Read the model definition and answer for the solid it produces. Units are mm, in the model's axes. Face numbers are marked on the shaded views. A direction names the side the tool comes from. Coordinates: 2 decimals unless noted, no trailing zeros. Write each loop counter-clockwise with the first axis right and the second up, starting at its lowest first coordinate (ties: lowest second). Pieces come first, ordered by that corner, then holes. Notation, with made-up numbers: (-14, 82) - (33, 82) arc R13 ccw to (33, 95) - close; hole circle Ø11 at (11, 88.25). An arc over 180 degrees is marked (long way). Use a Markdown table: item, result.
from build123d import *

# Parameters (mm, degrees)
SKETCH1_R           = 1.65
BOSS_EXTRUDE1_DEPTH = 2
BOSS_EXTRUDE2_DEPTH = 18
SKETCH3_W           = 13
SKETCH3_H           = 10
BOSS_EXTRUDE3_DEPTH = 10
SKETCH4_R           = 3.25
CUT_EXTRUDE1_DEPTH  = 10
CIRPATTERN1_COUNT   = 3


with BuildPart() as part:
    # Sketch1 → Boss-Extrude1 (new body)
    with BuildSketch(Plane(origin=(0, 0, 0), x_dir=(1, 0, 0), z_dir=(0, 1, 0))):
        with BuildLine():
            Line((14.5, 47.85133227), (48.690469351, -11.36829778))
            ThreePointArc((48.690469351, -11.36829778), (43.301270189, -25), (34.190469351, -36.48303449))
            Line((34.190469351, -36.48303449), (-34.190469351, -36.48303449))
            ThreePointArc((-34.190469351, -36.48303449), (-43.301270189, -25), (-48.690469351, -11.36829778))
            Line((-48.690469351, -11.36829778), (-14.5, 47.85133227))
            ThreePointArc((-14.5, 47.85133227), (0, 50), (14.5, 47.85133227))
        make_face()
        with Locations(Location((0, 45, 0), (0, 0, 270))):
            Circle(SKETCH1_R, mode=Mode.SUBTRACT)
        with Locations(Location((38.97114317, -22.5, 0), (0, 0, 270))):
            Circle(SKETCH1_R, mode=Mode.SUBTRACT)
        with Locations(Location((-38.97114317, -22.5, 0), (0, 0, 270))):
            Circle(SKETCH1_R, mode=Mode.SUBTRACT)
    extrude(amount=BOSS_EXTRUDE1_DEPTH)

    # Sketch2 → Boss-Extrude2 (add)
    with BuildSketch(Plane(origin=(0, 2, 0), x_dir=(1, 0, 0), z_dir=(0, 1, 0))):
        with BuildLine():
            Line((-14.5, 47.85133227), (-14.5, 8.371578903))
            Line((-14.5, 8.371578903), (-48.690469351, -11.36829778))
            ThreePointArc((-48.690469351, -11.36829778), (-48.443824061, -12.377233549), (-48.176274578, -13.380828366))
            Line((-48.176274578, -13.380828366), (-12.5, 7.216878365))
            Line((-12.5, 7.216878365), (-12.5, 48.412291828))
            ThreePointArc((-12.5, 48.412291828), (-13.502913349, 48.142199068), (-14.5, 47.85133227))
        make_face()
        with BuildLine():
            Line((14.5, 47.85133227), (14.5, 8.371578903))
            Line((14.5, 8.371578903), (48.690469351, -11.36829778))
            ThreePointArc((48.690469351, -11.36829778), (48.443824061, -12.377233549), (48.176274578, -13.380828366))
            Line((48.176274578, -13.380828366), (12.5, 7.216878365))
            Line((12.5, 7.216878365), (12.5, 48.412291828))
            ThreePointArc((12.5, 48.412291828), (13.502913349, 48.142199068), (14.5, 47.85133227))
        make_face()
        with BuildLine():
            Line((-34.190469351, -36.48303449), (0, -16.743157806))
            Line((0, -16.743157806), (34.190469351, -36.48303449))
            ThreePointArc((34.190469351, -36.48303449), (34.940910712, -35.764965519), (35.676274578, -35.031463461))
            Line((35.676274578, -35.031463461), (0, -14.43375673))
            Line((0, -14.43375673), (-35.676274578, -35.031463461))
            ThreePointArc((-35.676274578, -35.031463461), (-34.940910712, -35.764965519), (-34.190469351, -36.48303449))
        make_face()
    extrude(amount=BOSS_EXTRUDE2_DEPTH)

    # Sketch3 → Boss-Extrude3 (add)
    with BuildSketch(Plane(origin=(31.595234675, 0, -18.241517245), x_dir=(-0.5000000000000003, 0, -0.8660254037844386), z_dir=(0.8660254037844385, 0, -0.5000000000000002))):
        with Locations((0, 7)):
            Rectangle(SKETCH3_W, SKETCH3_H)
    boss_extrude3 = extrude(amount=-BOSS_EXTRUDE3_DEPTH)

    # Sketch4 → Cut-Extrude1 (cut)
    with BuildSketch(Plane(origin=(31.595234675, 0, -18.241517245), x_dir=(-0.5000000000000003, 0, -0.8660254037844385), z_dir=(0.8660254037844385, 0, -0.5000000000000003))):
        with Locations((0, 5)):
            Circle(SKETCH4_R)
    cut_extrude1 = extrude(amount=-CUT_EXTRUDE1_DEPTH, mode=Mode.SUBTRACT)

    # CirPattern1: Boss-Extrude3, Cut-Extrude1 ×3 about axis
    cirpattern1_axis = Axis((0, 0, 0), (0, 1, 0))
    add([boss_extrude3.rotate(cirpattern1_axis, i * 360 / CIRPATTERN1_COUNT) for i in range(1, CIRPATTERN1_COUNT)])
    add([cut_extrude1.rotate(cirpattern1_axis, i * 360 / CIRPATTERN1_COUNT) for i in range(1, CIRPATTERN1_COUNT)], mode=Mode.SUBTRACT)


solid = part.part
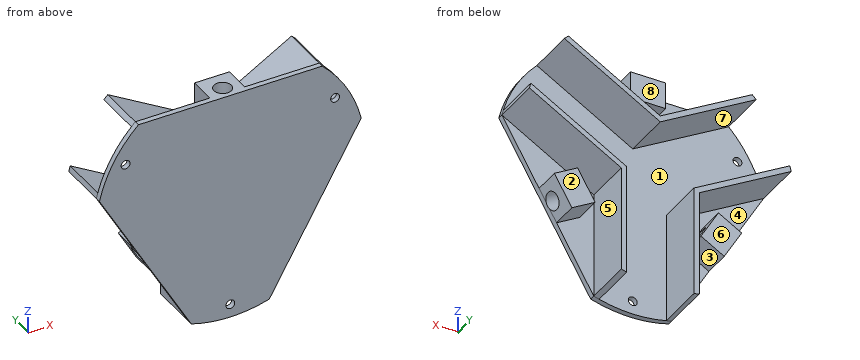
(1) For the marked faces 4, 5, 6, 7 and 8, determine the directions among +Z, -Z, +X, -X, +Y, -Y from which every point of the face is accessible in a straight line to the end or side of a thin tool.
Report:
| item | result |
|---|---|
| face 4 | +Y |
| face 5 | -Z, +Y |
| face 6 | -Z, -X, +Y |
| face 7 | -X, +Y |
| face 8 | +Z, +Y |
(2) A cutting plane is placed at C-C, the plane x = 9.5. Write down the section's boundary in (y, z).
Report:
| item | result |
|---|---|
| outline | (0, -49.09) - (2, -49.09) - (2, 19.92) - (20, 19.92) - (20, 22.23) - (2, 22.23) - (2, 36.48) - (0, 36.48) - close |
(3) A cutting plane is placed at D-D, the plane y = 6.75. Count the separate pieces of the cut face and the enclosed holes in it, and give its area (3 significant figures).
Report:
| item | result |
|---|---|
| separate pieces | 9 |
| enclosed holes | 0 |
| area | 710 mm² |
(4) A cutting plane is placed at B-B, the plane z = -45. Write down the section's boundary in (x, y).
Report:
| item | result |
|---|---|
| outline | (-16.15, 0) - (-1.65, 0) - (-1.65, 2) - (-12.5, 2) - (-12.5, 20) - (-14.5, 20) - (-14.5, 2) - (-16.15, 2) - close; (1.65, 0) - (16.15, 0) - (16.15, 2) - (14.5, 2) - (14.5, 20) - (12.5, 20) - (12.5, 2) - (1.65, 2) - close |
(5) A cutting plane is placed at A-A, the plane z = 22.5. Write down the section's boundary in (x, y).
Report:
| item | result |
|---|---|
| outline | (-44.65, 0) - (-40.62, 0) - (-40.62, 2) - (-44.65, 2) - close; (-37.32, 0) - (37.32, 0) - (37.32, 2) - (13.97, 2) - (13.97, 20) - (9.97, 20) - (9.97, 2) - (-9.97, 2) - (-9.97, 20) - (-13.97, 20) - (-13.97, 2) - (-37.32, 2) - close; (40.62, 0) - (44.65, 0) - (44.65, 2) - (40.62, 2) - close |
(6) Each of these flat-tipped pins is pushed along its axis until it touches: P1, Ø5, axis at x = 11.5, z = 4.5, coming from the -Y side; P2, Ø10.5, axis at x = 26, z = -25.5, coming from the +Y side; P3, Ø4, axis at x = -33.5, y = 17, coming from the +Z side; P4, Ø1.5, axis at y = 3.5, z = 12.5, coming from the -X side. Where does it stop, or does it pass through?
Report:
| item | result |
|---|---|
| P1 | stops at y = 0 |
| P2 | stops at y = 12 |
| P3 | stops at z = 36.48 |
| P4 | stops at x = -48.6 |
(7) Straight lines are drawn through the part: L1, parallel to Z at x = 28, y = 5.25; L2, parallel to X at y = 1.4, z = 22.5; L3, parallel to X at y = 18.5, z = -16. For each, find the intervals that lie inside material, in ascending order.
Report:
| item | result |
|---|---|
| L1 | z = -23.67 to -19.91, -12.42 to -8.66, -0.58 to 1.73, 30.6 to 32.91 |
| L2 | x = -44.65 to -40.62, -37.32 to 37.32, 40.62 to 44.65 |
| L3 | x = -14.5 to -12.5, 12.5 to 14.5 |
(8) The mould has two halves that part along Z. Classify the marked faces 1, 2 and 3: pulls with the +Z half, pulls with the -Z half, needs draft (parallel to the pull), parting line crosses it, or undercut.
Report:
| item | result |
|---|---|
| face 1 | undercut |
| face 2 | needs draft |
| face 3 | pulls with the -Z half |
